```python
from build123d import *

# Parameters (mm, degrees)
ESQUISSE2_W             = 32
ESQUISSE2_H             = 43
BOSS_EXTRU_1_DEPTH      = 32.5
ESQUISSE3_R             = 0.7
ENL_V_MAT_EXTRU_1_DEPTH = 43.12481454
ESQUISSE4_R             = 4.5
BOSS_EXTRU_2_DEPTH      = 1.5
ESQUISSE5_R             = 9.5
ESQUISSE5_R_2           = 0.004347537
BOSS_EXTRU_3_DEPTH      = 2
ESQUISSE6_R             = 0.8
ENL_V_MAT_EXTRU_2_DEPTH = 2
ESQUISSE7_R             = 4.5
BOSS_EXTRU_4_DEPTH      = 1
ENL_V_MAT_EXTRU_4_DEPTH = 43.12481454
ENL_V_START             = -5
ENL_V_MAT_EXTRU_5_DEPTH = 22


with BuildPart() as part:
    # Esquisse2 → Boss.-Extru.1 (new body)
    with BuildSketch(Plane.XY):
        Rectangle(ESQUISSE2_W, ESQUISSE2_H)
    extrude(amount=BOSS_EXTRU_1_DEPTH)

    # Esquisse3 → Enlèv. mat.-Extru.1 (cut, through all)
    with BuildSketch(Plane.XY.offset(32.5)):
        with Locations((-13.5, -18.5)):
            Circle(ESQUISSE3_R)
        with Locations((-13.5, 8.5)):
            Circle(ESQUISSE3_R)
        with Locations(Location((13.5, 8.5, 0), (0, 0, 180))):
            Circle(ESQUISSE3_R)
        with Locations(Location((13.5, -18.5, 0), (0, 0, 180))):
            Circle(ESQUISSE3_R)
    extrude(amount=-ENL_V_MAT_EXTRU_1_DEPTH, mode=Mode.SUBTRACT)

    # Esquisse4 → Boss.-Extru.2 (add)
    with BuildSketch(Plane.XY.offset(32.5)):
        with Locations((0, 9.5)):
            Circle(ESQUISSE4_R)
    boss_extru_2 = extrude(amount=BOSS_EXTRU_2_DEPTH)

    # Esquisse5 → Boss.-Extru.3 (add)
    with BuildSketch(Plane.XY.offset(34)):
        with Locations((0, 9.5)):
            Circle(ESQUISSE5_R)
        with Locations((-2.77085543, 1.343871271)):
            Circle(ESQUISSE5_R_2, mode=Mode.SUBTRACT)
    boss_extru_3 = extrude(amount=BOSS_EXTRU_3_DEPTH)

    # Esquisse6 → Enlèv. mat.-Extru.2 (cut)
    with BuildSketch(Plane.XY.offset(36)):
        with Locations((-7, 9.5)):
            Circle(ESQUISSE6_R)
        with Locations((-4.949747468, 14.449747468)):
            Circle(ESQUISSE6_R)
        with Locations((0, 16.5)):
            Circle(ESQUISSE6_R)
        with Locations((4.949747468, 14.449747468)):
            Circle(ESQUISSE6_R)
        with Locations((7, 9.5)):
            Circle(ESQUISSE6_R)
        with Locations((4.949747468, 4.550252532)):
            Circle(ESQUISSE6_R)
        with Locations((0, 2.5)):
            Circle(ESQUISSE6_R)
        with Locations((-4.949747468, 4.550252532)):
            Circle(ESQUISSE6_R)
    enl_v_mat_extru_2 = extrude(amount=-ENL_V_MAT_EXTRU_2_DEPTH, mode=Mode.SUBTRACT)

    # Esquisse7 → Boss.-Extru.4 (add)
    with BuildSketch(Plane.XY.offset(36)):
        with Locations((0, 9.5)):
            Circle(ESQUISSE7_R)
    boss_extru_4 = extrude(amount=BOSS_EXTRU_4_DEPTH)

    # Esquisse10 → Enlèv. mat.-Extru.4 (cut, through all)
    with BuildSketch(Plane.XY.offset(32.5)):
        with BuildLine():
            add(Edge.make_bspline(
                [(-16, 11.510544327), (-15.437884563, 17.715114653), (-10.032085652, 21.5)],
                knots=[0.188379191, 0.188379191, 0.188379191, 1, 1, 1], degree=2))
            Line((-10.032085652, 21.5), (-16, 21.5))
            Line((-16, 21.5), (-16, 11.510544327))
        make_face()
        with BuildLine():
            Line((16, 21.5), (10.032085652, 21.5))
            add(Edge.make_bspline(
                [(16, 11.510544327), (15.437884563, 17.715114653), (10.032085652, 21.5)],
                knots=[0.188379191, 0.188379191, 0.188379191, 1, 1, 1], degree=2))
            Line((16, 11.510544327), (16, 21.5))
        make_face()
    extrude(amount=-ENL_V_MAT_EXTRU_4_DEPTH, mode=Mode.SUBTRACT)

    # Esquisse14 → Enlèv. mat.-Extru.5 (cut)
    with BuildSketch(Plane.ZY.offset(16).offset(ENL_V_START)):
        with BuildLine():
            Line((0, -19.5), (0, -21.5))
            Line((0, -21.5), (2, -21.5))
            ThreePointArc((2, -21.5), (0.585786438, -20.914213562), (0, -19.5))
        make_face()
        with BuildLine():
            Line((32.5, -19.5), (32.5, -21.5))
            Line((32.5, -21.5), (30.5, -21.5))
            ThreePointArc((30.5, -21.5), (31.914213562, -20.914213562), (32.5, -19.5))
        make_face()
    extrude(amount=-ENL_V_MAT_EXTRU_5_DEPTH, mode=Mode.SUBTRACT)

    # Symétrie1: Boss.-Extru.2, Boss.-Extru.3, Enlèv. mat.-Extru.2, Boss.-Extru.4 across plane
    add(boss_extru_2.mirror(Plane.XY.offset(16.25)))
    add(boss_extru_3.mirror(Plane.XY.offset(16.25)))
    add(enl_v_mat_extru_2.mirror(Plane.XY.offset(16.25)), mode=Mode.SUBTRACT)
    add(boss_extru_4.mirror(Plane.XY.offset(16.25)))


solid = part.part
```
Build history of the part. All positions in model axes, mm. A direction names the side the tool comes from. Round coordinates to 2 decimals unless told otherwise and drop trailing zeros. Write each loop counter-clockwise with the first axis right and the second up, starting at its lowest first coordinate (ties: lowest second). Pieces come first, ordered by that corner, then holes. Notation, with made-up numbers: (31, 1.5) -> (84, 1.5) arc R24 cw to (84, 19.5) -> close; hole circle Ø5 at (73.5, 23.5). An arc over 180 degrees is marked (long way). Put each result on its own line as item: value.
Item 1: Slice it at D-D, the plane z = 24. Count the separate pieces of the cut face and the enclosed holes in it, plus the area to 3 significant figures.
Here are the results:
separate pieces: 1
enclosed holes: 4
area: 1,330 mm^2
Item 2: Flat gauge pins, fed straight in: P1, Ø10, axis at x = 11.5, y = -14, coming from the +Z side; P2, Ø1, axis at x = 4.95, y = 14.45, coming from the -Z side; P3, Ø2, axis at x = -4.95, y = 14.45, coming from the -Z side; P4, Ø0.8, axis at x = 13.5, y = -18.5, coming from the -Z side. Where does each tip first touch, or does it go through?
Here are the results:
P1: stops at z = 32.5
P2: stops at z = 0
P3: stops at z = -3.5
P4: passes through
Item 3: Wall check: probe 1 along Z at (x, y) = (8, 14); probe 2 along Y at (x, z) = (0, -1.95); probe 3 along X at (y, z) = (9, 7.5). Give the ranges that are in metal, low to high. Write a range as from..to.
Here are the results:
probe 1: z = -3.5..-1.5, 0..32.5, 34..36
probe 2: y = 0..1.7, 3.3..15.7, 17.3..19
probe 3: x = -16..-13.99, -13.01..13.01, 13.99..16
Item 4: Slice it at A-A, the plane y = -18.5. Give the cut face in (x, z), plus the area to 3 significant figures.
Here are the results:
outline: (-16, 0) -> (-14.2, 0) -> (-14.2, 32.5) -> (-16, 32.5) -> close; (-12.8, 0) -> (12.8, 0) -> (12.8, 32.5) -> (-12.8, 32.5) -> close; (14.2, 0) -> (16, 0) -> (16, 32.5) -> (14.2, 32.5) -> close
area: 949 mm^2
Item 5: Slice it at C-C, the plane y = 2.5. Give the cut face in (x, z).
Here are the results:
outline: (-16, 0) -> (16, 0) -> (16, 32.5) -> (-16, 32.5) -> close; (-6.42, -3.5) -> (-0.8, -3.5) -> (-0.8, -1.5) -> (-6.42, -1.5) -> close; (-6.42, 34) -> (-0.8, 34) -> (-0.8, 36) -> (-6.42, 36) -> close; (0.8, -3.5) -> (6.42, -3.5) -> (6.42, -1.5) -> (0.8, -1.5) -> close; (0.8, 34) -> (6.42, 34) -> (6.42, 36) -> (0.8, 36) -> close
Item 6: Two-plate mould, pull along Y, no slides. Class faces 4 (the face through (-5.054, 15.243, -2.514)), 5 (the face through (5.11, 17.51, -2.49)), 6 (the face through (0, 10, -4.5)): pulls with the +Y half, pulls with the -Y half, needs draft (parallel to the pull), parting line crosses it, or undercut.
Here are the results:
face 4: undercut
face 5: parting line crosses it
face 6: needs draft
Item 7: Slice it at B-B, the plane x = -7. Give the cut face in (y, z).
Here are the results:
outline: (-21.5, 2) arc R2 ccw to (-19.5, 0) -> (21.5, 0) -> (21.5, 32.5) -> (-19.5, 32.5) arc R2 ccw to (-21.5, 30.5) -> close; (3.08, -3.5) -> (8.7, -3.5) -> (8.7, -1.5) -> (3.08, -1.5) -> close; (3.08, 34) -> (8.7, 34) -> (8.7, 36) -> (3.08, 36) -> close; (10.3, -3.5) -> (15.92, -3.5) -> (15.92, -1.5) -> (10.3, -1.5) -> close; (10.3, 34) -> (15.92, 34) -> (15.92, 36) -> (10.3, 36) -> close
Item 8: Tool access for faces 1 (the face through (-0.59, 13.96, 36.49)), 2 (the face through (-0.59, 13.96, 33.24)), 3 (the face through (4.15, 14.48, -2.51)): list every direction of +Z, -Z, +X, -X, +Y, -Y with a clear straight run to the whole face (end or side of a thin tool).
Here are the results:
face 1: +Z
face 2: none
face 3: -Z
